from build123d import *

# Parameters (mm, degrees)
SKETCH1_R           = 12.5
SKETCH1_R_2         = 7
BOSS_EXTRUDE1_DEPTH = 5
CUT_EXTRUDE1_REACH  = 20.371
SKETCH2_R           = 1.525


with BuildPart() as part:
    # Sketch1 → Boss-Extrude1 (new body)
    with BuildSketch(Plane.XY):
        Circle(SKETCH1_R)
        Circle(SKETCH1_R_2, mode=Mode.SUBTRACT)
    extrude(amount=BOSS_EXTRUDE1_DEPTH)

    # Sketch2 → Cut-Extrude1 (cut, up to next)
    with BuildSketch(Plane.XY.offset(5), mode=Mode.PRIVATE) as cut_extrude1_sk1:
        with Locations((0, 9.75)):
            Circle(SKETCH2_R)
    cut_extrude1_tool1 = extrude(cut_extrude1_sk1.sketch, amount=-CUT_EXTRUDE1_REACH, mode=Mode.PRIVATE) & part.part
    # Sketch2 → Cut-Extrude1 (cut, up to next)
    with BuildSketch(Plane.XY.offset(5), mode=Mode.PRIVATE) as cut_extrude1_sk2:
        with Locations((8.443747687, -4.875)):
            Circle(SKETCH2_R)
    cut_extrude1_tool2 = extrude(cut_extrude1_sk2.sketch, amount=-CUT_EXTRUDE1_REACH, mode=Mode.PRIVATE) & part.part
    # Sketch2 → Cut-Extrude1 (cut, up to next)
    with BuildSketch(Plane.XY.offset(5), mode=Mode.PRIVATE) as cut_extrude1_sk3:
        with Locations((-8.443747687, -4.875)):
            Circle(SKETCH2_R)
    cut_extrude1_tool3 = extrude(cut_extrude1_sk3.sketch, amount=-CUT_EXTRUDE1_REACH, mode=Mode.PRIVATE) & part.part
    add(cut_extrude1_tool1.solids().sort_by_distance((0, 9.75, 5))[0], mode=Mode.SUBTRACT)
    add(cut_extrude1_tool2.solids().sort_by_distance((8.443748, -4.875, 5))[0], mode=Mode.SUBTRACT)
    add(cut_extrude1_tool3.solids().sort_by_distance((-8.443748, -4.875, 5))[0], mode=Mode.SUBTRACT)


solid = part.part
Could you check a few things on this model? Use its own coordinates, in mm. Give positions to 0.01 mm unless a question says otherwise; leave off trailing zeros. Loops run counter-clockwise (first coordinate to the right, second up) from the corner with the lowest first, then second, coordinate; pieces in that order, holes last. Notation, with made-up numbers: M 82.5,-12.5 L 140.5,-12.5 A34 cw 140.5,22.5 Z; hole C 37.25,23.5 d5. An arc over 180 degrees is marked long. Answer as a JSON object with one key per item and string values.
Q1. For P1, Ø3, axis at x = 6.5, z = 2, coming from the +Y side; P2, Ø3, axis at y = 6.5, z = 3, coming from the -X side; P3, Ø1.5, axis at x = 8, z = 1, coming from the +Y side, each with a flat end and sliding along its axis, tell me the tip position at first contact or that it passes through.
Values found:
{"P1": "stops at y = 11.46", "P2": "stops at x = -11.46", "P3": "stops at y = 10.18"}
Q2. Suppose I cut it at C-C, the plane y = -4. List the corners of the cut face in (x, z) for me, plus the area to 3 significant figures.
Values found:
{"outline": "M -11.84,0 L -9.69,0 L -9.69,5 L -11.84,5 Z; M -7.19,0 L -5.74,0 L -5.74,5 L -7.19,5 Z; M 5.74,0 L 7.19,0 L 7.19,5 L 5.74,5 Z; M 9.69,0 L 11.84,0 L 11.84,5 L 9.69,5 Z", "area": "36.0 mm²"}
Q3. Suppose I cut it at D-D, the plane x = -4.5. List the corners of the cut face in (y, z) for me.
Values found:
{"outline": "M -11.66,0 L -5.36,0 L -5.36,5 L -11.66,5 Z; M 5.36,0 L 11.66,0 L 11.66,5 L 5.36,5 Z"}
Q4. If I drill on probe 1 along Y at (x, z) = (0, 2.75) (3 decimals); probe 2 along X at (y, z) = (-4.5, 0.25); probe 3 along X at (y, z) = (-5.25, 4.3), over which ranges is the centre line in solid material (lowest first)? Write a range as [from, to].
Values found:
{"probe 1": "y = [-12.5, -7], [7, 8.225], [11.275, 12.5]", "probe 2": "x = [-11.66, -9.92], [-6.97, -5.36], [5.36, 6.97], [9.92, 11.66]", "probe 3": "x = [-11.34, -9.92], [-6.97, -4.63], [4.63, 6.97], [9.92, 11.34]"}
Q5. Suppose I cut it at B-B, the plane x = 0. List the corners of the cut face in (y, z) for me (3 decimals).
Values found:
{"outline": "M -12.5,0 L -7,0 L -7,5 L -12.5,5 Z; M 7,0 L 8.225,0 L 8.225,5 L 7,5 Z; M 11.275,0 L 12.5,0 L 12.5,5 L 11.275,5 Z"}
Q6. If we mould it in two halves opening along X, with no side actions, what happens to faces 1 (the cylindrical face through (11.923, 3.755, 2.465)), 2 (the cylindrical face through (-0.2, 11.26, 2.54)), 3 (the flat face through (5.4, -5.4, 5)), 4 (the cylindrical face through (6.92, -4.81, 2.54))? For each: pulls with the +X half, pulls with the -X half, needs draft (parallel to the pull), parting line crosses it, or undercut.
Values found:
{"face 1": "parting line crosses it", "face 2": "undercut", "face 3": "needs draft", "face 4": "undercut"}
Q7. Suppose I cut it at A-A, the plane y = 0. List the corners of the cut face in (x, z) for me, plus the area to 3 significant figures.
Values found:
{"outline": "M -12.5,0 L -7,0 L -7,5 L -12.5,5 Z; M 7,0 L 12.5,0 L 12.5,5 L 7,5 Z", "area": "55.0 mm²"}
